Read the model definition and answer for the solid it produces. Units are mm, in the model's axes. A direction names the side the tool comes from. Coordinates: 2 decimals unless noted, no trailing zeros. Order: outer loops, then holes, each group sorted by start corner. A loop starts at its lowest first (then second) coordinate and runs counter-clockwise, first axis right, second up. Notation, with made-up numbers: (37, -29.75) -> (82, -29.75) arc R21 cw to (82, -13.75) -> close; hole circle Ø11 at (-34, -37). An arc over 180 degrees is marked (long way). Use CSV: the item, a comma, the result in double quotes.
```python
from build123d import *

# Parameters (mm, degrees)
F0_W     = 2
F0_H     = 1000
F1_DEPTH = 90
F0_W_2   = 648
F0_W_3   = 50.688
F0_H_2   = 6.08256
F0_R     = 4.05504
F0_W_4   = 45
F0_H_3   = 170
F2_DEPTH = 2


with BuildPart() as f1:
    # F0 (on Front) → F1 (new body)
    with BuildSketch(Plane.XZ):
        with Locations((-199, 300)):
            Rectangle(F0_W, F0_H)
    extrude(amount=-F1_DEPTH)

    # F0 (on Front) → F2 (join)
    with BuildSketch(Plane.XZ):
        with Locations((126, 300)):
            Rectangle(F0_W_2, F0_H)
        with Locations((-3.208926, -17.236022)):
            Rectangle(F0_W_3, F0_H_2, mode=Mode.SUBTRACT)
        with BuildLine():
            Line((-28.636116, -9.734198), (-28.636116, -1.015862))
            Line((-28.636116, -1.015862), (-23.364564, 7.702474))
            Line((-23.364564, 7.702474), (-19.309524, 7.702474))
            ThreePointArc((-19.309524, 7.702474), (-16.442178, 6.51478), (-15.254484, 3.647434))
            Line((-15.254484, 3.647434), (-15.254484, -9.734198))
            Line((-15.254484, -9.734198), (-16.673748, -9.734198))
            ThreePointArc((-16.673748, -9.734198), (-20.728788, -13.789238), (-24.783828, -9.734198))
            Line((-24.783828, -9.734198), (-28.636116, -9.734198))
        make_face(mode=Mode.SUBTRACT)
        with Locations((1.649359, -9.818369)):
            Circle(F0_R, mode=Mode.SUBTRACT)
        with Locations((11.326316, -9.814243)):
            Circle(F0_R, mode=Mode.SUBTRACT)
        Polygon((22.609892, -10.377738), (-12.615537, 9.709673), (-6.589313, 20.277302), (28.636116, 0.18989), align=None, mode=Mode.SUBTRACT)
        with Locations((-72.5, 645)):
            Rectangle(F0_W_4, F0_H_3, mode=Mode.SUBTRACT)
    extrude(amount=-F2_DEPTH)


solid = f1.part
```
Item 1: A tool of negligible diameter and unlimited length cuts with its end or side. For faces 1 (the flat face through (-198, 45, 293)), 2 (the flat face through (10.777, 0.986, 10.374)), 3 (the flat face through (120, 0, 307)), from which of +Z, -Z, +X, -X, +Y, -Y can it reach the whole face along a straight path? Write none if from no direction.
Return value:
face 1,"+Z, -Z, +X, +Y"
face 2,"+Y, -Y"
face 3,"+Z, -Z, +X, -X, -Y"
Item 2: Find section A-A, the plane z = 246. Give the vertices of the cut face in (x, y).
Return value:
outline,"(-200, 0) -> (450, 0) -> (450, 2) -> (-198, 2) -> (-198, 90) -> (-200, 90) -> close"
Item 3: This flat-tipped pin is pushed along its axis until it touches: P1, Ø1.5, axis at x = 360, z = 533.5, coming from the +Y side. Where does it stop, or does it pass through?
Return value:
P1,"stops at y = 2"
Item 4: Straight lines are drawn through the part: line 1 along Y through (x, z) = (-1.5, 400); line 2 along X through (y, z) = (58.5, 683). For each, find the intervals that lie inside material, in ascending order.
Return value:
line 1,"y = 0 to 2"
line 2,"x = -200 to -198"
Item 5: The mould has two halves that part along Z. Classify faces 4 (the flat face through (123, 1, 800)), 5 (the flat face through (121, 2, 307)), 6 (the flat face through (5.244, 0.986, -0.475)), 7 (the flat face through (123, 1, -200)): +Z half, -Z half, draft (parallel to the pull), parting line (faces both ways), or undercut.
Return value:
face 4,"+Z half"
face 5,"draft"
face 6,"undercut"
face 7,"-Z half"
Item 6: Find section B-B, the plane x = 231.5. Give the vertices of the cut face in (y, z), then the cut area to 3 significant figures.
Return value:
outline,"(0, -200) -> (2, -200) -> (2, 800) -> (0, 800) -> close"
area,"2,000 mm^2"
Item 7: Find section C-C, the plane y = 71. Give the vertices of the cut face in (x, z).
Return value:
outline,"(-200, -200) -> (-198, -200) -> (-198, 800) -> (-200, 800) -> close"
